Read the model definition and answer for the solid it produces. Units are mm, in the model's axes. Round coordinates to 2 decimals unless told otherwise and drop trailing zeros. Write each loop counter-clockwise with the first axis right and the second up, starting at its lowest first coordinate (ties: lowest second). Pieces come first, ordered by that corner, then holes. Notation, with made-up numbers: (-29.5, -39) -> (10.5, -39) arc R23 cw to (10.5, -12) -> close; hole circle Ø1 at (75.5, 77.5). An arc over 180 degrees is marked (long way). Return JSON: item names as keys, results as strings. Group by question number.
(1) A cutting plane is placed at C-C on x = 3.5. Give the vertices of the cut face in (y, z), then the cut area to 3 significant figures.
(2) A cutting plane is placed at B-B on z = 0. Give the vertices of the cut face in (x, y).
(3) Given pin 1 (1.5 mm diameter, centred on x = 8, y = -2, fed in from +Z); pin 2 (2.5 mm diameter, centred on y = -13.47, z = 13.47, fed in from +X); pin 3 (6 mm diameter, centred on y = 0, z = 0, fed in from -X); pin 4 (4 mm diameter, centred on x = 7, z = -9, fed in from -Y), each flat-ended and moving along its own axis, determine where each tip first touches the part or whether it passes through.
(4) The mould has two halves that part along Y. Classify faces 1 (the cylindrical face through (5.07, -19.255, 14.864)), 2 (the flat face through (7.2, -2, 2)), 3 (the cylindrical face through (5.07, 19.233, 14.951)), 4 (the cylindrical face through (3.55, 1.49, 4.72)): released by +Y, released by -Y, zero draft, split by the parting line, or undercut.
(5) A cutting plane is placed at D-D on z = -13. Give the vertices of the cut face in (x, y), then the cut area to 3 significant figures.
(6) A cutting plane is placed at A-A on y = 0. Give the vertices of the cut face in (x, z), then the cut area to 3 significant figures.
(7) Straight lines are drawn through the part: line 1 (Y direction, x = 4.25, z = -13.5); line 2 (Y direction, x = 8.5, z = -13); line 3 (Z direction, x = 7.25, y = 13). For each, find the intervals that lie inside material, in ascending order.
```python
from build123d import *

# Parameters (mm, degrees)
SKETCH_1_R          = 25
EXTRUDE_1_DEPTH     = 10
SKETCH_3_R          = 2.45
CUT_EXTRUDE_1_DEPTH = 37.742346142
SKETCH_5_R          = 4.95
CUT_EXTRUDE_2_DEPTH = 7.2
SKETCH_6_R          = 2
CUT_EXTRUDE_3_DEPTH = 37.742346142
SKETCH_7_R          = 1.65
CUT_EXTRUDE_4_DEPTH = 37.742346142
CUT_EXTRUDE_5_DEPTH = 37.742346142


with BuildPart() as part:
    # ｽｹｯﾁ1 → ﾎﾞｽ - 押し出し1 (new body)
    with BuildSketch(Plane(origin=(0, 0, 0), x_dir=(0, 0, -1), z_dir=(1, 0, 0))):
        Circle(SKETCH_1_R)
    extrude(amount=EXTRUDE_1_DEPTH)

    # ｽｹｯﾁ3 → ｶｯﾄ - 押し出し1 (cut, through all)
    with BuildSketch(Plane(origin=(10, 0, 0), x_dir=(0, 0, -1), z_dir=(1, 0, 0))):
        Circle(SKETCH_3_R)
    extrude(amount=-CUT_EXTRUDE_1_DEPTH, mode=Mode.SUBTRACT)

    # ｽｹｯﾁ5 → ｶｯﾄ - 押し出し2 (cut)
    with BuildSketch(Plane.ZY):
        Circle(SKETCH_5_R)
    extrude(amount=-CUT_EXTRUDE_2_DEPTH, mode=Mode.SUBTRACT)

    # ｽｹｯﾁ6 → ｶｯﾄ - 押し出し3 (cut, through all)
    with BuildSketch(Plane(origin=(10, 0, 0), x_dir=(0, 0, -1), z_dir=(1, 0, 0))):
        with Locations((-19.05, 0)):
            Circle(SKETCH_6_R)
        with Locations(Location((19.05, 0, 0), (0, 0, 180))):
            Circle(SKETCH_6_R)
    extrude(amount=-CUT_EXTRUDE_3_DEPTH, mode=Mode.SUBTRACT)

    # ｽｹｯﾁ7 → ｶｯﾄ - 押し出し4 (cut, through all)
    with BuildSketch(Plane(origin=(10, 0, 0), x_dir=(0, 0, -1), z_dir=(1, 0, 0))):
        with Locations((13.470384182, 13.470384182)):
            Circle(SKETCH_7_R)
        with Locations((13.470384182, -13.470384182)):
            Circle(SKETCH_7_R)
        with Locations((-13.470384182, -13.470384182)):
            Circle(SKETCH_7_R)
        with Locations((-13.470384182, 13.470384182)):
            Circle(SKETCH_7_R)
    extrude(amount=-CUT_EXTRUDE_4_DEPTH, mode=Mode.SUBTRACT)

    # ｽｹｯﾁ8 → ｶｯﾄ - 押し出し5 (cut, through all)
    with BuildSketch(Plane(origin=(10, 0, 0), x_dir=(0, 0, -1), z_dir=(1, 0, 0))):
        with BuildLine():
            ThreePointArc((-17.67766953, 17.67766953), (-14.907460792, 19.244231323), (-11.726124041, 19.158974214))
            ThreePointArc((-11.726124041, 19.158974214), (-3.5e-08, 17.401594613), (11.726123974, 19.158974194))
            ThreePointArc((11.726123974, 19.158974194), (14.907460759, 19.244231332), (17.67766953, 17.67766953))
            ThreePointArc((17.67766953, 17.67766953), (0, 25), (-17.67766953, 17.67766953))
        make_face()
        with BuildLine():
            ThreePointArc((-11.726124073, -19.158974224), (-14.90746082, -19.244231316), (-17.677669546, -17.677669513))
            ThreePointArc((-17.677669546, -17.677669513), (-4.3e-08, -25), (17.677669486, -17.677669573))
            ThreePointArc((17.677669486, -17.677669573), (14.9074607, -19.244231346), (11.726123917, -19.158974177))
            ThreePointArc((11.726123917, -19.158974177), (-8.1e-08, -17.401594613), (-11.726124073, -19.158974224))
        make_face()
    extrude(amount=-CUT_EXTRUDE_5_DEPTH, mode=Mode.SUBTRACT)


solid = part.part
```
Checks:
{
 "1": {"outline": "(-19.16, -11.73) arc R5.95 ccw to (-17.68, -17.68) arc R25 ccw to (17.68, -17.68) arc R5.95 ccw to (19.16, -11.73) arc R40 cw to (19.16, 11.73) arc R5.95 ccw to (17.68, 17.68) arc R25 ccw to (-17.68, 17.68) arc R5.95 ccw to (-19.16, 11.73) arc R40 cw to start; hole circle Ø3.3 at (-13.47, -13.47); hole circle Ø3.3 at (-13.47, 13.47); hole circle Ø9.9 at (0, 0); hole circle Ø4 at (0, -19.05); hole circle Ø4 at (0, 19.05); hole circle Ø3.3 at (13.47, -13.47); hole circle Ø3.3 at (13.47, 13.47)", "area": "1,520 mm^2"},
 "2": {"outline": "(0, -17.4) -> (10, -17.4) -> (10, -2.45) -> (7.2, -2.45) -> (7.2, -4.95) -> (0, -4.95) -> close; (0, 4.95) -> (7.2, 4.95) -> (7.2, 2.45) -> (10, 2.45) -> (10, 17.4) -> (0, 17.4) -> close"},
 "3": {"pin 1": "stops at z = 24.97", "pin 2": "passes through", "pin 3": "stops at x = 7.2", "pin 4": "stops at y = -18.94"},
 "4": {"face 1": "released by -Y", "face 2": "undercut", "face 3": "released by +Y", "face 4": "undercut"},
 "5": {"outline": "(0, -19.4) -> (10, -19.4) -> (10, -15.05) -> (0, -15.05) -> close; (0, -11.89) -> (10, -11.89) -> (10, 11.89) -> (0, 11.89) -> close; (0, 15.05) -> (10, 15.05) -> (10, 19.4) -> (0, 19.4) -> close", "area": "325 mm^2"},
 "6": {"outline": "(0, -25) -> (10, -25) -> (10, -21.05) -> (0, -21.05) -> close; (0, -17.05) -> (10, -17.05) -> (10, -2.45) -> (7.2, -2.45) -> (7.2, -4.95) -> (0, -4.95) -> close; (0, 4.95) -> (7.2, 4.95) -> (7.2, 2.45) -> (10, 2.45) -> (10, 17.05) -> (0, 17.05) -> close; (0, 21.05) -> (10, 21.05) -> (10, 25) -> (0, 25) -> close", "area": "335 mm^2"},
 "7": {"line 1": "y = -19.42 to -15.12, -11.82 to 11.82, 15.12 to 19.42", "line 2": "y = -19.4 to -15.05, -11.89 to 11.89, 15.05 to 19.4", "line 3": "z = -21.35 to -15.05, -11.89 to 11.89, 15.05 to 21.35"}
}
